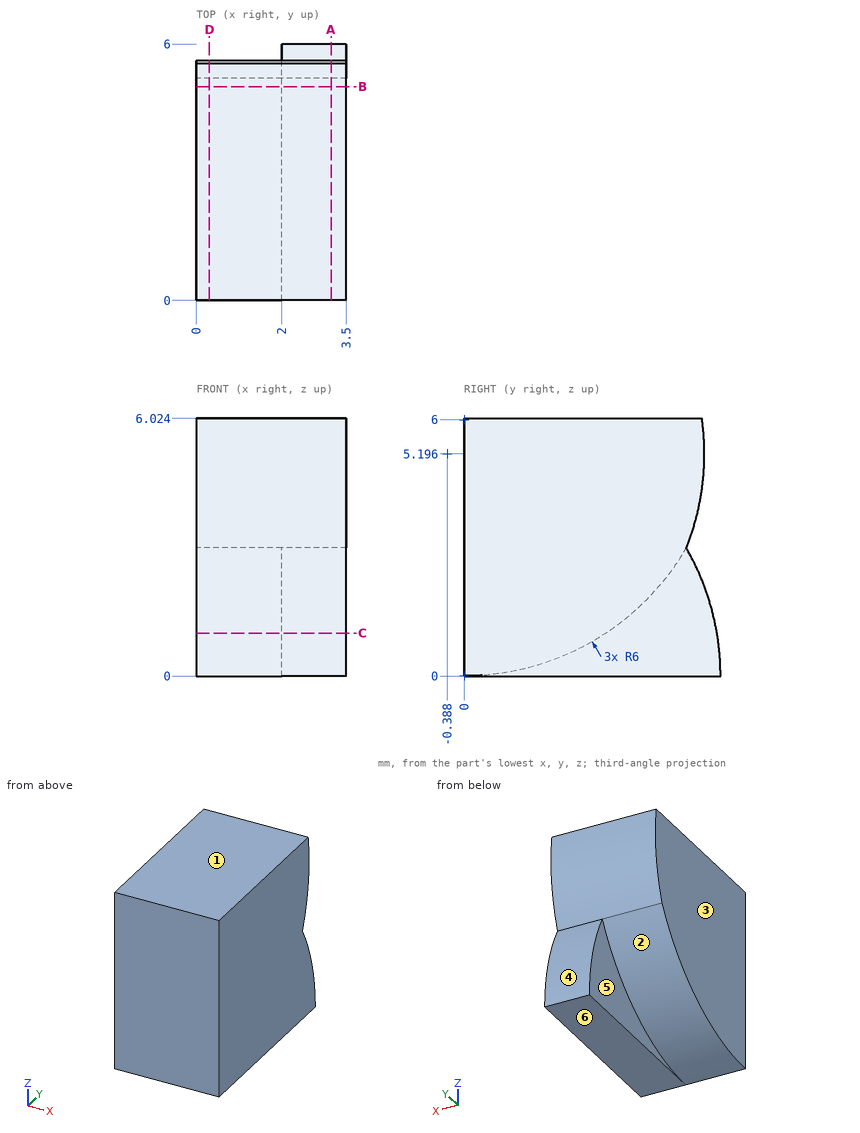
Design review of the part shown in the three views and the two pictorial views. Dimensions are in mm from the part's minimum x, y and z. A direction names the side the tool comes from. Round coordinates to 2 decimals unless told otherwise and drop trailing zeros. Loops run counter-clockwise (first coordinate to the right, second up) from the corner with the lowest first, then second, coordinate; pieces in that order, holes last. Notation, with made-up numbers: (-6.75, 22.5) - (39.25, 22.5) arc R16 ccw to (39.25, 31.5) - close; hole circle Ø2 at (53.25, 54). An arc over 180 degrees is marked (long way). Use one line per item in the form item = value.
1) Tool access review of the marked faces 5 and 6: name each direction out of +Z, -Z, +X, -X, +Y, -Y from which nothing blocks a thin tool from reaching the whole face with its end or side.
Solutions:
face_5 = -Z, -X, +Y
face_6 = -Z, +X, -X, +Y, -Y
2) We need section A-A on x = 3.15. Write out the cut boundary in (y, z) (1 decimal), then the cut area to 3 significant figures.
Solutions:
outline = (0, 0) - (6, 0) arc R6 ccw to (5.2, 3) arc R6 ccw to (5.6, 6) - (0, 6) - close
area = 33.9 mm2
3) We need section B-B on y = 5. Write out the cut boundary in (x, z).
Solutions:
outline = (0, 2.68) - (2, 2.68) - (2, 0) - (3.5, 0) - (3.5, 6.02) - (0, 6.02) - close
4) We need section D-D on x = 0.3. Write out the cut boundary in (y, z) (1 decimal).
Solutions:
outline = (0, 0) arc R6 ccw to (5.2, 3) arc R6 ccw to (5.6, 6) - (0, 6) - close
5) Mouldability with a two-part tool opening along Z and no side actions: class the marked faces 1, 2, 3 and 4 as pulls with the +Z half, pulls with the -Z half, needs draft (parallel to the pull), parting line crosses it, or undercut.
Solutions:
face_1 = pulls with the +Z half
face_2 = pulls with the -Z half
face_3 = needs draft
face_4 = undercut
6) We need section C-C on z = 1. Write out the cut boundary in (x, y).
Solutions:
outline = (0, 0) - (3.5, 0) - (3.5, 5.92) - (2, 5.92) - (2, 3.32) - (0, 3.32) - close
7) Wall thickness on probe 1 along Y at (x, z) = (2.8, 2.5) (1 decimal); probe 2 along Y at (x, z) = (2.45, 5.75); probe 3 along Z at (x, y) = (0.2, 2.55) (1 decimal): over which ranges is each line inside the solid? List them lowest first.
Solutions:
probe_1 = 0 to 5.5
probe_2 = 0 to 5.59
probe_3 = 0.6 to 6
